The listing builds one solid part. Answer for the finished solid, in the listing's coordinates (mm). A direction names the side the tool comes from. Round coordinates to 2 decimals unless told otherwise and drop trailing zeros. Loops run counter-clockwise (first coordinate to the right, second up) from the corner with the lowest first, then second, coordinate; pieces in that order, holes last. Notation, with made-up numbers: (32.5, 46.5) - (52.5, 46.5) arc R30 cw to (52.5, 80.5) - close; hole circle Ø6 at (36.5, 71). An arc over 180 degrees is marked (long way). One line per item, written item: value.
```python
from build123d import *

# Parameters (mm, degrees)
EXTRUDE_1_DEPTH           = 120
HOLE_WIZARD_1_D           = 9
HOLE_WIZARD_1_CBORE_D     = 15
HOLE_WIZARD_1_CBORE_DEPTH = 9
CUT_EXTRUDE_1_REACH       = 172.22
SKETCH_6_R                = 2.1
CHAMFER_2_SIZE            = 2.5
CHAMFER_3_SIZE            = 2
CHAMFER_3_SIZE2           = 2.400003543
CHAMFER_4_SIZE            = 2


with BuildPart() as part:
    # 草图1 → 凸台-拉伸1 (new body)
    with BuildSketch(Plane.XY):
        Polygon((0, 0), (51, 0), (120, -10.8), (120, -18.5), (78, -17.1875), (78, -13.2175), (62, -13.2175), (62, -16.6875), (24, -15.5), (24, -18.5), (0, -18.5), align=None)
    extrude(amount=EXTRUDE_1_DEPTH)

    # 孔1 (through all)
    with Locations(Plane(origin=(0, -18.5, 0), x_dir=(-1, 0, 0), z_dir=(0, -1, 0))):
        with Locations((-12.5, -20), (-12.5, -60), (-12.5, -100)):
            CounterBoreHole(HOLE_WIZARD_1_D / 2, HOLE_WIZARD_1_CBORE_D / 2, HOLE_WIZARD_1_CBORE_DEPTH)

    # 切除-拉伸1: up to this plane
    cut_extrude_1_end = Plane(origin=(51, 0, 120), z_dir=(-0.15463894699101186, -0.9879710502203549, 0))
    # 草图6 → 切除-拉伸1 (cut, up to the surface)
    with BuildSketch(Plane.XZ.offset(13.2175), mode=Mode.PRIVATE) as cut_extrude_1_sk1:
        with Locations((70, 100)):
            Circle(SKETCH_6_R)
    cut_extrude_1_tool1 = split(extrude(cut_extrude_1_sk1.sketch, amount=-CUT_EXTRUDE_1_REACH, mode=Mode.PRIVATE), bisect_by=cut_extrude_1_end, keep=Keep.BOTH, mode=Mode.PRIVATE)
    add(cut_extrude_1_tool1.solids().sort_by_distance((70, -13.2175, 100))[0], mode=Mode.SUBTRACT)
    # 草图6 → 切除-拉伸1 (cut, up to the surface)
    with BuildSketch(Plane.XZ.offset(13.2175), mode=Mode.PRIVATE) as cut_extrude_1_sk2:
        with Locations((70, 60)):
            Circle(SKETCH_6_R)
    cut_extrude_1_tool2 = split(extrude(cut_extrude_1_sk2.sketch, amount=-CUT_EXTRUDE_1_REACH, mode=Mode.PRIVATE), bisect_by=cut_extrude_1_end, keep=Keep.BOTH, mode=Mode.PRIVATE)
    add(cut_extrude_1_tool2.solids().sort_by_distance((70, -13.2175, 60))[0], mode=Mode.SUBTRACT)
    # 草图6 → 切除-拉伸1 (cut, up to the surface)
    with BuildSketch(Plane.XZ.offset(13.2175), mode=Mode.PRIVATE) as cut_extrude_1_sk3:
        with Locations((70, 20)):
            Circle(SKETCH_6_R)
    cut_extrude_1_tool3 = split(extrude(cut_extrude_1_sk3.sketch, amount=-CUT_EXTRUDE_1_REACH, mode=Mode.PRIVATE), bisect_by=cut_extrude_1_end, keep=Keep.BOTH, mode=Mode.PRIVATE)
    add(cut_extrude_1_tool3.solids().sort_by_distance((70, -13.2175, 20))[0], mode=Mode.SUBTRACT)

    # 倒角2
    chamfer_2_edges = [part.edges().sort_by_distance(p)[0] for p in [
        (120, -14.65, 0),
        (0, -9.25, 0),
        (120, -14.65, 120),
        (0, -9.25, 120),
    ]]
    chamfer(chamfer_2_edges, length=CHAMFER_2_SIZE)

    # 倒角3
    chamfer_3_edges = [part.edges().sort_by_distance(p)[0] for p in [
        (120, -10.8, 60),
    ]]
    chamfer_3_side = [part.faces().sort_by_distance(p)[0] for p in [
        (120, -14.65, 60),
    ]]
    chamfer(chamfer_3_edges, length=CHAMFER_3_SIZE, length2=CHAMFER_3_SIZE2, reference=chamfer_3_side[0])

    # 倒角4
    chamfer_4_edges = [part.edges().sort_by_distance(p)[0] for p in [
        (0, 0, 60),
    ]]
    chamfer(chamfer_4_edges, length=CHAMFER_4_SIZE)


solid = part.part
```
1) For a pull along Z with two mould halves and no side action, classify faces 4 (the cylindrical face through (16.66, -4.68, 61.72)), 5 (the flat face through (48, -9, 0)), 6 (the flat face through (48, -9, 120)), 7 (the flat face through (120, -16, 59)) as released by +Z, released by -Z, zero draft, split by the parting line, or undercut.
Final values:
face 4: undercut
face 5: released by -Z
face 6: released by +Z
face 7: zero draft
2) A cutting plane is placed at D-D on z = 40. Give the vertices of the cut face in (x, y), and give its area (3 significant figures).
Final values:
outline: (0, -18.5) - (24, -18.5) - (24, -15.5) - (62, -16.69) - (62, -13.22) - (78, -13.22) - (78, -17.19) - (120, -18.5) - (120, -12.8) - (117.63, -10.43) - (51, 0) - (2, 0) - (0, -2) - close
area: 1,640 mm2
3) Consider L1, parallel to Z at x = 12.5, y = -12.75; L2, parallel to X at y = -13.5, z = 60; L3, parallel to Z at x = 15.5, y = -14. Determine where each line is inside the solid, lowest interval first.
Final values:
L1: 0 to 12.5, 27.5 to 52.5, 67.5 to 92.5, 107.5 to 120
L2: 0 to 5, 20 to 62, 78 to 120
L3: 0 to 13.13, 26.87 to 53.13, 66.87 to 93.13, 106.87 to 120
4) A cutting plane is placed at B-B on z = 100. Give the vertices of the cut face in (x, y), and give its area (3 significant figures).
Final values:
outline: (0, -18.5) - (5, -18.5) - (5, -9.5) - (8, -9.5) - (8, 0) - (2, 0) - (0, -2) - close; (17, -9.5) - (20, -9.5) - (20, -18.5) - (24, -18.5) - (24, -15.5) - (62, -16.69) - (62, -13.22) - (67.9, -13.22) - (67.9, -2.65) - (51, 0) - (17, 0) - close; (72.1, -13.22) - (78, -13.22) - (78, -17.19) - (120, -18.5) - (120, -12.8) - (117.63, -10.43) - (72.1, -3.3) - close
area: 1,380 mm2
5) Each of these flat-tipped pins is pushed along its axis until it touches: pin 1 Ø3 at (y, z) = (-10, 96.5) entering from +X; pin 2 Ø8 at (x, z) = (12.5, 60) entering from -Y; pin 3 Ø8 at (x, z) = (70, 50) entering from -Y; pin 4 Ø7.5 at (x, z) = (9, 99.5) entering from -Y. Where does it stop, or does it pass through?
Final values:
pin 1: x = 118.7
pin 2: through
pin 3: y = -13.22
pin 4: y = -9.5
6) A cutting plane is placed at A-A on x = 12.5. Give the vertices of the cut face in (y, z).
Final values:
outline: (-18.5, 0) - (0, 0) - (0, 15.5) - (-9.5, 15.5) - (-9.5, 12.5) - (-18.5, 12.5) - close; (-18.5, 27.5) - (-9.5, 27.5) - (-9.5, 24.5) - (0, 24.5) - (0, 55.5) - (-9.5, 55.5) - (-9.5, 52.5) - (-18.5, 52.5) - close; (-18.5, 67.5) - (-9.5, 67.5) - (-9.5, 64.5) - (0, 64.5) - (0, 95.5) - (-9.5, 95.5) - (-9.5, 92.5) - (-18.5, 92.5) - close; (-18.5, 107.5) - (-9.5, 107.5) - (-9.5, 104.5) - (0, 104.5) - (0, 120) - (-18.5, 120) - close
7) For faces 1 (the cylindrical face through (68.334, -7.99, 58.722)), 2 (the flat face through (24, -17, 59)), 3 (the flat face through (7.6, -9.5, 59.9)), determine the directions among +Z, -Z, +X, -X, +Y, -Y from which every point of the face is accessible in a straight line to the end or side of a thin tool.
Final values:
face 1: +Y, -Y
face 2: +Z, -Z, -Y
face 3: -Y
8) A cutting plane is placed at C-C on y = -5.5. Give the vertices of the cut face in (x, z), and give its area (3 significant figures).
Final values:
outline: (0, 2.5) - (2.5, 0) - (86.14, 0) - (86.14, 120) - (2.5, 120) - (0, 117.5) - close; hole circle Ø9 at (12.5, 20); hole circle Ø9 at (12.5, 60); hole circle Ø9 at (12.5, 100); hole circle Ø4.2 at (70, 20); hole circle Ø4.2 at (70, 60); hole circle Ø4.2 at (70, 100)
area: 10,100 mm2
